Source: CAD feature listing. Evaluate the final solid. Frame: model axes, mm. A direction names the side the tool comes from. Coordinates: 2 decimals unless noted, no trailing zeros. Order: outer loops, then holes, each group sorted by start corner. A loop starts at its lowest first (then second) coordinate and runs counter-clockwise, first axis right, second up. Notation, with made-up numbers: (65.25, -21) -> (109.25, -21) arc R10 ccw to (109.25, -8) -> close; hole circle Ø3 at (57, 39). An arc over 180 degrees is marked (long way). Put each result on its own line as item: value.
Autodesk Fusion 360 part; units mm, degrees
sketch "Sketch1" plane through (0, 0, 0) normal (0, 0, 1) x (1, 0, 0)
  line L0 (100, 0) -> (100, 25)
  line L1 (100, 25) -> (12.5683, 25)
  line L2 (12.5683, 25) -> (0.9567, 20.1903)
  arc A0 (0, 20) -> (0.9567, 20.1903) centre (0, 22.5) ccw
  line L3 (0, 0) -> (100, 0) construction
  line L4 (0, 0) -> (0, 20) construction
  line L5 (100, 20) -> (0, 20) construction
  line L6 (100, 0) -> (100, -25) construction
  line L7 (100, -25) -> (12.5683, -25) construction
  line L8 (12.5683, -25) -> (0.9567, -20.1903) construction
  arc A1 (0.9567, -20.1903) -> (0, -20) centre (0, -22.5) ccw construction
  arc A2 (-0.9567, 20.1903) -> (0, 20) centre (0, 22.5) ccw
  line L9 (-12.5683, 25) -> (-0.9567, 20.1903)
  line L10 (-100, 25) -> (-12.5683, 25)
  line L11 (-100, 0) -> (-100, 25)
  line L12 (-100, 0) -> (-100, -25) construction
  line L13 (-100, -25) -> (-12.5683, -25) construction
  line L14 (-12.5683, -25) -> (-0.9567, -20.1903) construction
  arc A3 (0, -20) -> (-0.9567, -20.1903) centre (0, -22.5) ccw construction
  line L15 (-100, 0) -> (100, 0)
  dimension "Notch_Radius" = 2.5
  dimension "Notch_Height" = 5
  dimension "Bar_Diameter" = 50
  dimension "Bar_Length" = 200
  dimension "Notch_Theta" = 135
revolve "Revolve1" add sketch "Sketch1" angle 360 about axis through (-100, 0, 0) along (1, 0, 0)
1. Cut plane B-B on x = -3. Output: boundary loops of the cut face in (y, z).
Numbers:
outline: circle Ø42.07 at (0, 0)
2. First-contact query: pin 1 (5 mm diameter, centred on x = -36, z = -5.5, fed in from -Y); pin 2 (10 mm diameter, centred on x = 51.5, z = 7, fed in from -Y); pin 3 (8 mm diameter, centred on x = -25.5, z = -16.5, fed in from -Y). Flat tips, straight axial feed; report the tip coordinate or a pass-through.
Numbers:
pin 1: stops at y = -24.82
pin 2: stops at y = -24.92
pin 3: stops at y = -21.65
3. Set-up query: faces 1 (the flat face through (-100, 0, 0)), 2 (the conical face through (-1.683, -4.442, 20.004)). Return all of +Z, -Z, +X, -X, +Y, -Y with unobstructed straight access to the full face (end or side cutting, diameter ignored); none if empty.
Numbers:
face 1: +Z, -Z, -X, +Y, -Y
face 2: none
4. Cut plane A-A on x = 86. Output: boundary loops of the cut face in (y, z).
Numbers:
outline: circle Ø50 at (0, 0)
5. Ray query, line 1 along X through (y, z) = (-10, 18); line 2 along X through (y, z) = (-16, -15); line 3 along Z through (x, y) = (-10, 3.5). Return the intervals inside material, ascending.
Numbers:
line 1: x = -100 to -1.92, 1.92 to 100
line 2: x = -100 to -5.16, 5.16 to 100
line 3: z = -23.68 to 23.68
